```python
from build123d import *

# Parameters (mm, degrees)
F0_W     = 18.7
F0_H     = 12
F1_DEPTH = 3.2
F3_R     = 3.3
F4_DEPTH = 2.8
F2_R     = 2


with BuildPart() as f1:
    # F0 (on Top) → F1 (new body)
    with BuildSketch(Plane.XY):
        Rectangle(F0_W, F0_H)
    extrude(amount=F1_DEPTH)

    # F3 (on face) → F4 (cut)
    with BuildSketch(Plane(origin=(0, 0, 0), x_dir=(1, 0, 0), z_dir=(0, 0, -1))):
        with Locations((0, -2)):
            Circle(F3_R)
    extrude(amount=-F4_DEPTH, mode=Mode.SUBTRACT)

    # F6: sweep along a path in F5
    with BuildLine(Plane.YZ) as f6_path:
        Line((-3.5, 3.2), (-2.4647238196, 7.0637033052))
    # F2 (on face) → F6 (sweep)
    with BuildSketch(Plane.XY.offset(3.2)):
        with Locations((0, -3.5)):
            Circle(F2_R)
    sweep(path=f6_path.line)


solid = f1.part
```
The model under review builds one solid part; all positions refer to its coordinate system, in mm. Round coordinates to 2 decimals unless told otherwise and drop trailing zeros. Order: outer loops, then holes, each group sorted by start corner. A loop starts at its lowest first (then second) coordinate and runs counter-clockwise, first axis right, second up. Notation, with made-up numbers: (61.5, 80) -> (66.5, 80) arc R18 cw to (66.5, 94) -> close; hole circle Ø6 at (-14.75, 45.5). An arc over 180 degrees is marked (long way). Use a Markdown table: item, result.
Q1. For line 1 (Y direction, x = 0, z = 2.1); line 2 (X direction, y = 2, z = 2.1); line 3 (Z direction, x = 0.5, y = 1.25), list the stretches that pass through material, from the lowest coordinate up.
Values:
| item | result |
|---|---|
| line 1 | y = -6 to -1.3, 5.3 to 6 |
| line 2 | x = -9.35 to -3.3, 3.3 to 9.35 |
| line 3 | z = 2.8 to 3.2 |
Q2. We need section C-C on y = 0. Write out the cut boundary in (x, z), then the cut area to 3 significant figures.
Values:
| item | result |
|---|---|
| outline | (-9.35, 0) -> (-2.62, 0) -> (-2.62, 2.8) -> (2.62, 2.8) -> (2.62, 0) -> (9.35, 0) -> (9.35, 3.2) -> (-9.35, 3.2) -> close |
| area | 45.1 mm^2 |
Q3. Clearance check with a flat-ended pin moving along its axis: P1, Ø3.5, axis at x = -4, y = -3, coming from the +Z side. State where the tip first meets the part, or that it passes through.
Values:
| item | result |
|---|---|
| P1 | stops at z = 3.2 |
Q4. We need section B-B on x = -6.75. Write out the cut boundary in (y, z).
Values:
| item | result |
|---|---|
| outline | (-6, 0) -> (6, 0) -> (6, 3.2) -> (-6, 3.2) -> close |
Q5. We need section A-A on y = 2. Write out the cut boundary in (x, z).
Values:
| item | result |
|---|---|
| outline | (-9.35, 0) -> (-3.3, 0) -> (-3.3, 2.8) -> (3.3, 2.8) -> (3.3, 0) -> (9.35, 0) -> (9.35, 3.2) -> (-9.35, 3.2) -> close |
Q6. Mouldability with a two-part tool opening along Y and no side actions: class faces 1 (the flat face through (2, -1, 0)), 2 (the flat face through (0, 2, 2.8)), 3 (the cylindrical face through (-0.43, -1.27, 1.38)), 4 (the flat face through (0, -6, 2)) as +Y half, -Y half, draft (parallel to the pull), parting line (faces both ways), or undercut.
Values:
| item | result |
|---|---|
| face 1 | draft |
| face 2 | undercut |
| face 3 | undercut |
| face 4 | -Y half |
